Design review of the part built by this model. Coordinates are the model's own, in mm. Face numbers are marked on the shaded views. A direction names the side the tool comes from. Coordinates: 2 decimals unless noted, no trailing zeros. Loops run counter-clockwise (first coordinate to the right, second up) from the corner with the lowest first, then second, coordinate; pieces in that order, holes last. Notation, with made-up numbers: (-18.5, 65.5) -> (-4.5, 65.5) arc R26 cw to (-4.5, 93.5) -> close; hole circle Ø9 at (23.25, 82.25). An arc over 180 degrees is marked (long way). Answer in a Markdown table with one row per item.
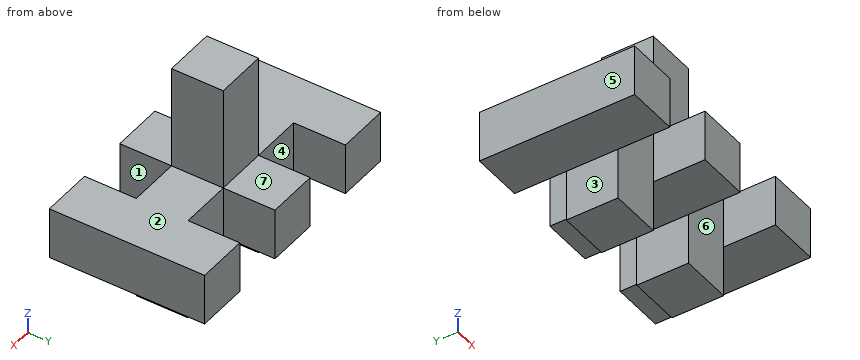
```python
from build123d import *

# Parameters (mm, degrees)
F0_W     = 25.4
F0_H     = 25.4
F1_DEPTH = 25.4
F2_W     = 25.4
F2_H     = 25.4
F3_DEPTH = 50.8
F4_W     = 25.4
F4_H     = 25.4
F5_DEPTH = 25.4


with BuildPart() as f1:
    # F0 (on Top) → F1 (new body)
    with BuildSketch(Plane.XY):
        Polygon((63.5, -12.7), (63.5, 12.7), (38.1, 12.7), (12.7, 12.7), (-12.7, 12.7), (-38.1, 12.7), (-63.5, 12.7), (-63.5, -12.7), (-38.1, -12.7), (-12.7, -12.7), (12.7, -12.7), (38.1, -12.7), align=None)
        with Locations((50.8, 25.4)):
            Rectangle(F0_W, F0_H)
        with Locations((50.8, -25.4)):
            Rectangle(F0_W, F0_H)
        with Locations((0, 25.4)):
            Rectangle(F0_W, F0_H)
        with Locations((0, -25.4)):
            Rectangle(F0_W, F0_H)
        with Locations((-50.8, 25.4)):
            Rectangle(F0_W, F0_H)
        with Locations((-50.8, -25.4)):
            Rectangle(F0_W, F0_H)
    extrude(amount=F1_DEPTH)

    # F2 (on face) → F3 (join)
    with BuildSketch(Plane.XY.offset(25.4)):
        Rectangle(F2_W, F2_H)
    extrude(amount=F3_DEPTH)

    # F4 (on face) → F5 (join)
    with BuildSketch(Plane(origin=(0, 0, 0), x_dir=(1, 0, 0), z_dir=(0, 0, -1))):
        with Locations((-25.4, 0)):
            Rectangle(F4_W, F4_H)
        with Locations((25.4, 0)):
            Rectangle(F4_W, F4_H)
    extrude(amount=F5_DEPTH)


solid = f1.part
```
(1) Take a section at C-C on x = -4.5. Give the boundary of the cut face in (y, z), and give its area (3 significant figures).
Evaluation:
| item | result |
|---|---|
| outline | (-38.1, 0) -> (38.1, 0) -> (38.1, 25.4) -> (12.7, 25.4) -> (12.7, 76.2) -> (-12.7, 76.2) -> (-12.7, 25.4) -> (-38.1, 25.4) -> close |
| area | 3,230 mm² |
(2) Take a section at D-D on y = 4. Give the boundary of the cut face in (x, z).
Evaluation:
| item | result |
|---|---|
| outline | (-63.5, 0) -> (-38.1, 0) -> (-38.1, -25.4) -> (-12.7, -25.4) -> (-12.7, 0) -> (12.7, 0) -> (12.7, -25.4) -> (38.1, -25.4) -> (38.1, 0) -> (63.5, 0) -> (63.5, 25.4) -> (12.7, 25.4) -> (12.7, 76.2) -> (-12.7, 76.2) -> (-12.7, 25.4) -> (-63.5, 25.4) -> close |
(3) Take a section at A-A on z = -14. Give the boundary of the cut face in (x, y), and give its area (3 significant figures).
Evaluation:
| item | result |
|---|---|
| outline | (-38.1, -12.7) -> (-12.7, -12.7) -> (-12.7, 12.7) -> (-38.1, 12.7) -> close; (12.7, -12.7) -> (38.1, -12.7) -> (38.1, 12.7) -> (12.7, 12.7) -> close |
| area | 1,290 mm² |
(4) For pin 1 (1.5 mm diameter, centred on y = 9.5, z = 48, fed in from -X); pin 2 (20.5 mm diameter, centred on x = 24.5, z = -12.5, fed in from +Y); pin 3 (12.5 mm diameter, centred on y = 1.5, z = 62.5, fed in from +X), all flat-tipped, find the tip position at first contact; note any pin that passes through.
Evaluation:
| item | result |
|---|---|
| pin 1 | stops at x = -12.7 |
| pin 2 | stops at y = 12.7 |
| pin 3 | stops at x = 12.7 |
(5) Take a section at B-B on z = 8.5. Give the boundary of the cut face in (x, y).
Evaluation:
| item | result |
|---|---|
| outline | (-63.5, -38.1) -> (-38.1, -38.1) -> (-38.1, -12.7) -> (-12.7, -12.7) -> (-12.7, -38.1) -> (12.7, -38.1) -> (12.7, -12.7) -> (38.1, -12.7) -> (38.1, -38.1) -> (63.5, -38.1) -> (63.5, 38.1) -> (38.1, 38.1) -> (38.1, 12.7) -> (12.7, 12.7) -> (12.7, 38.1) -> (-12.7, 38.1) -> (-12.7, 12.7) -> (-38.1, 12.7) -> (-38.1, 38.1) -> (-63.5, 38.1) -> close |
(6) To check wall thickness, follow probe 1 along X at (y, z) = (22, 6.5); probe 2 along Z at (x, y) = (-15.5, 9.5); probe 3 along Z at (x, y) = (-46, 5). State the ranges of each line that lie inside material, in increasing order.
Evaluation:
| item | result |
|---|---|
| probe 1 | x = -63.5 to -38.1, -12.7 to 12.7, 38.1 to 63.5 |
| probe 2 | z = -25.4 to 25.4 |
| probe 3 | z = 0 to 25.4 |
(7) Draft analysis for pull direction X (two halves, no side actions). For the marked faces 5, 6 and 7, state which applies: pulls with the +X half, pulls with the -X half, needs draft (parallel to the pull), parting line crosses it, or undercut.
Evaluation:
| item | result |
|---|---|
| face 5 | pulls with the -X half |
| face 6 | undercut |
| face 7 | needs draft |
(8) Tool access review of the marked faces 1, 2, 3 and 4: name each direction out of +Z, -Z, +X, -X, +Y, -Y from which nothing blocks a thin tool from reaching the whole face with its end or side.
Evaluation:
| item | result |
|---|---|
| face 1 | +Z, -Z, -Y |
| face 2 | +Z, +X, +Y, -Y |
| face 3 | -Z, -X, +Y, -Y |
| face 4 | +Z, -Z, +Y |
